Geometry check sheet. Reference: the model listing, model coordinates, mm. Round coordinates to 2 decimals unless told otherwise and drop trailing zeros. Loops run counter-clockwise (first coordinate to the right, second up) from the corner with the lowest first, then second, coordinate; pieces in that order, holes last. Notation, with made-up numbers: (75, 67) - (112, 67) arc R27 ccw to (112, 97) - close; hole circle Ø9 at (83, 62.25). An arc over 180 degrees is marked (long way). Answer as CSV lines item,"result". Start each with the question number.
1) Cross-section at A-A on x = 0.75. Record the boundary of the cut face in (y, z), and give its area (3 significant figures).
2) Depth check by flat-ended pin: P1, Ø0.6, axis at x = 15, y = 0, coming from the +Z side. Enter the tip coordinate at first touch or a pass-through.
3) Cross-section at B-B on y = -18.5. Record the boundary of the cut face in (x, z).
4) Cross-section at C-C on z = 0.65. Record the boundary of the cut face in (x, y).
5) Thickness scan on line 1 along Y through (x, z) = (10.15, 0.1); line 2 along X through (y, z) = (-15, 0.35); line 3 along Z through (x, y) = (16.25, -8). Record the ranges inside material, lowest first.
Autodesk Fusion 360 part; units mm, degrees
sketch "Esboço1" plane through (0, 0, 0) normal (0, 0, 1) x (1, 0, 0)
  line L0 (-2.54, 2.54) -> (17.78, 2.54)
  line L1 (17.78, 2.54) -> (17.78, -25.4)
  line L2 (17.78, -25.4) -> (-2.54, -25.4)
  line L3 (-2.54, -25.4) -> (-2.54, 2.54)
extrude "Extrusão1" add sketch "Esboço1" along normal blind 0.3
sketch "Esboço2" plane through (0, 0, 0) normal (0, 0, 1) x (1, 0, 0)
  line L0 (-1, -2) -> (16, -2)
  line L1 (16, -2) -> (16, -24)
  line L2 (16, -24) -> (-1, -24)
  line L3 (-1, -24) -> (-1, -2)
extrude "Extrusão2" add sketch "Esboço2" along normal blind 0.8
sketch "Esboço3" plane through (0, 0, 0.3) normal (0, 0, 1) x (-1, 0, 0)
  line L0 (1, 24) -> (1, 2)
  line L1 (1, 2) -> (-16, 2)
  line L2 (-16, 2) -> (-16, 24)
  line L3 (-16, 24) -> (1, 24)
  line L4 (2.54, 25.4) -> (-17.78, 25.4)
  line L5 (-17.78, 25.4) -> (-17.78, -2.54)
  line L6 (-17.78, -2.54) -> (2.54, -2.54)
  line L7 (2.54, -2.54) -> (2.54, 25.4)
  circle A0 centre (0, 0) radius 0.25
  circle A1 centre (-2.5, 0) radius 0.25
  curve A2
  circle A3 centre (-7.62, 0.0108) radius 0.25
  circle A4 centre (-10.15, 0) radius 0.25
  circle A5 centre (-12.7077, 0.0204) radius 0.25
  circle A6 centre (-15.239, 0.0204) radius 0.25
  dimension "d5" = 0.5
  dimension "d6" = 0.5
  dimension "d7" = 0.5
  dimension "d8" = 0.5
  dimension "d9" = 0.5
  dimension "d10" = 0.5
  dimension "d11" = 0.5
extrude "Extrusão3" cut sketch "Esboço3" against normal blind 0.05 contours A3 | A4 | A5 | A6
sketch "Esboço4" plane through (0, 0, 0.3) normal (0, 0, 1) x (-1, 0, 0)
  circle A0 centre (-12.7077, 0.0204) radius 0.25
  circle A1 centre (-10.15, 0) radius 0.25
  circle A2 centre (-15.239, 0.0204) radius 0.25
  circle A3 centre (-7.62, 0.0108) radius 0.25
  line L0 (1, 24) -> (1, 2)
  line L1 (1, 2) -> (-16, 2)
  line L2 (-16, 2) -> (-16, 24)
  line L3 (-16, 24) -> (1, 24)
  line L4 (2.54, 25.4) -> (-17.78, 25.4)
  line L5 (-17.78, 25.4) -> (-17.78, -2.54)
  line L6 (-17.78, -2.54) -> (2.54, -2.54)
  line L7 (2.54, -2.54) -> (2.54, 25.4)
  circle A4 centre (-5.0796, 0.0001) radius 0.25
  circle A5 centre (-2.54, 0) radius 0.25
  circle A6 centre (0, 0) radius 0.25
  dimension "d14" = 0.5
  dimension "d15" = 0.5
  dimension "d16" = 0.5
extrude "Extrusão4" cut sketch "Esboço4" against normal blind 0.05 contours A4 | A5 | A6
sketch "Esboço5" plane through (0, 0, 0.3) normal (0, 0, 1) x (-1, 0, 0)
  circle A0 centre (-5.0796, 0.0001) radius 0.25
  circle A1 centre (-2.54, 0) radius 0.25
  circle A2 centre (0, 0) radius 0.25
  circle A3 centre (-12.7077, 0.0204) radius 0.25
  circle A4 centre (-10.15, 0) radius 0.25
  circle A5 centre (-15.239, 0.0204) radius 0.25
  circle A6 centre (-7.62, 0.0108) radius 0.25
  line L0 (1, 24) -> (1, 2)
  line L1 (1, 2) -> (-16, 2)
  line L2 (-16, 2) -> (-16, 24)
  line L3 (-16, 24) -> (1, 24)
  line L4 (2.54, 25.4) -> (-17.78, 25.4)
  line L5 (-17.78, 25.4) -> (-17.78, -2.54)
  line L6 (-17.78, -2.54) -> (2.54, -2.54)
  line L7 (2.54, -2.54) -> (2.54, 25.4)
  circle A7 centre (0, 0) radius 0.1
  circle A8 centre (-2.54, 0) radius 0.1
  circle A9 centre (-5.0796, 0.0001) radius 0.1
  circle A10 centre (-7.62, 0.0108) radius 0.1
  circle A11 centre (-10.15, 0) radius 0.1
  circle A12 centre (-12.7077, 0.0204) radius 0.1
  circle A13 centre (-15.239, 0.0204) radius 0.1
  dimension "d19" = 0.2
  dimension "d20" = 0.2
  dimension "d21" = 0.2
  dimension "d22" = 0.2
  dimension "d23" = 0.2
  dimension "d24" = 0.2
  dimension "d25" = 0.2
extrude "Extrusão5" cut sketch "Esboço5" against normal blind 2 contours A7 | A8 | A9 | A10 | A11 | A12 | A13
Answer block:
1,outline,"(-25.4, 0) - (2.54, 0) - (2.54, 0.3) - (-2, 0.3) - (-2, 0.8) - (-24, 0.8) - (-24, 0.3) - (-25.4, 0.3) - close"
1,area,"19.4 mm^2"
2,P1,"stops at z = 0.3"
3,outline,"(-2.54, 0) - (17.78, 0) - (17.78, 0.3) - (16, 0.3) - (16, 0.8) - (-1, 0.8) - (-1, 0.3) - (-2.54, 0.3) - close"
4,outline,"(-1, -24) - (16, -24) - (16, -2) - (-1, -2) - close"
5,line 1,"y = -25.4 to -0.1, 0.1 to 2.54"
5,line 2,"x = -1 to 16"
5,line 3,"z = 0 to 0.3"
